Geometry check sheet. Reference: the model listing, model coordinates, mm. Give positions to 0.01 mm unless a question says otherwise; leave off trailing zeros. Write each loop counter-clockwise with the first axis right and the second up, starting at its lowest first coordinate (ties: lowest second). Pieces come first, ordered by that corner, then holes.
(1) Thickness scan on line 1 along Z through (x, y) = (-0.25, 42); line 2 along Z through (x, y) = (0.5, 23); line 3 along X through (y, z) = (202, 0.5). Record the ranges inside material, lowest first.
(2) Depth check by flat-ended pin: P1, Ø3, axis at x = 0.5, y = 23.5, coming from the -Z side; P2, Ø1, axis at x = -1, y = 235.5, coming from the -Z side; P3, Ø1.5, axis at y = 161.5, z = -2.5, coming from the -X side. Enter the tip coordinate at first touch or a pass-through.
(3) Cross-section at B-B (z = -2.25). Record the boundary of the cut face in (x, y), and give its area (3 significant figures).
(4) Cross-section at A-A (y = 245). Record the boundary of the cut face in (x, z), and give its area (3 significant figures).
```python
from build123d import *

# Parameters (mm, degrees)
SKETCH1_R              = 4
BOSS_EXTRUDE1_DEPTH    = 330
CUT_EXTRUDE1_START     = -4
CUT_EXTRUDE1_OUTLINE_W = 3.911370479
CUT_EXTRUDE1_OUTLINE_H = 4.081430066
CUT_EXTRUDE1_DEPTH     = 0.5


# Read off the part's stored shape, not the designer's step: Cut-Extrude1
with BuildPart() as part:
    # Sketch1 → Boss-Extrude1 (new body)
    with BuildSketch(Plane(origin=(0, 0, 0), x_dir=(1, 0, 0), z_dir=(0, 1, 0))):
        with Locations(Location((0, 0, 0), (0, 0, 270))):
            Circle(SKETCH1_R)
    extrude(amount=BOSS_EXTRUDE1_DEPTH)

    # Cut-Extrude1 outline → Cut-Extrude1 (cut)
    with BuildSketch(Plane.XY.offset(CUT_EXTRUDE1_START)):
        with Locations((-0.357855864, 223.902178758)):
            Rectangle(CUT_EXTRUDE1_OUTLINE_W, CUT_EXTRUDE1_OUTLINE_H)
        with Locations((-0.357855864, 323.902178758)):
            Rectangle(CUT_EXTRUDE1_OUTLINE_W, CUT_EXTRUDE1_OUTLINE_H)
        with Locations((-0.357855864, 123.902178758)):
            Rectangle(CUT_EXTRUDE1_OUTLINE_W, CUT_EXTRUDE1_OUTLINE_H)
        with Locations((-0.357855864, 23.902178758)):
            Rectangle(CUT_EXTRUDE1_OUTLINE_W, CUT_EXTRUDE1_OUTLINE_H)
    extrude(amount=CUT_EXTRUDE1_DEPTH, mode=Mode.SUBTRACT)


solid = part.part
```
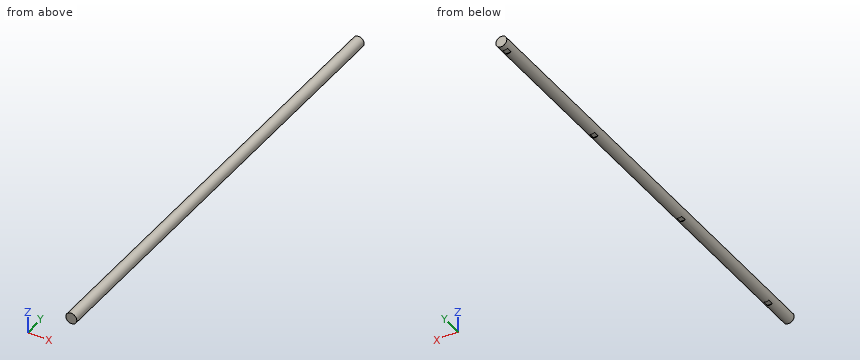
Reply:
1. line 1: z = -3.99 to 3.99
1. line 2: z = -3.5 to 3.97
1. line 3: x = -3.97 to 3.97
2. P1: stops at z = -3.67
2. P2: stops at z = -3.97
2. P3: stops at x = -3.6
3. outline: (-3.31, 0) - (3.31, 0) - (3.31, 330) - (-3.31, 330) - close
3. area: 2,180 mm2
4. outline: circle Ø8 at (0, 0)
4. area: 50.3 mm2
